Design review of the part built by this model. Coordinates are the model's own, in mm. A direction names the side the tool comes from. Give positions to 0.01 mm unless a question says otherwise; leave off trailing zeros. Write each loop counter-clockwise with the first axis right and the second up, starting at its lowest first coordinate (ties: lowest second). Pieces come first, ordered by that corner, then holes. Notation, with made-up numbers: (82.25, 76) -> (100.25, 76) arc R19 cw to (100.25, 102) -> close; hole circle Ø4 at (60, 42). An arc over 180 degrees is marked (long way). Answer as a JSON object with one key per item and string values.
```python
from build123d import *

# Parameters (mm, degrees)
SKETCH_1_R          = 2
SKETCH_1_W          = 20
SKETCH_1_H          = 50
EXTRUDE_1_DEPTH     = 3
FILLET_1_R          = 40
SKETCH_2_R          = 2
CUT_EXTRUDE_1_DEPTH = 10


with BuildPart() as part:
    # 草图1 → 凸台-拉伸1 (new body)
    # profile 1 of 3: a face of its own
    with BuildSketch(Plane.XY):
        Polygon((10, 36.547005384), (-10, 25), (10, 25), align=None)
    # profile 2 of 3: a face of its own
    with BuildSketch(Plane.XY):
        Polygon((20.980762114, 65.980762114), (30.980762114, 48.660254038), (-20.980762114, 18.660254038), (-30.980762114, 35.980762114), align=None)
        with Locations((0, 42.320508076)):
            Circle(SKETCH_1_R, mode=Mode.SUBTRACT)
        with Locations((17.320508076, 52.320508076)):
            Circle(SKETCH_1_R, mode=Mode.SUBTRACT)
        with Locations((-17.320508076, 32.320508076)):
            Circle(SKETCH_1_R, mode=Mode.SUBTRACT)
    # profile 3 of 3: a face of its own
    with BuildSketch(Plane.XY):
        Rectangle(SKETCH_1_W, SKETCH_1_H)
    extrude(amount=EXTRUDE_1_DEPTH)

    # 圆角1
    # the kernel refuses this fillet: 40 mm, written as the material it adds along each edge
    with BuildSketch(Plane(origin=(10, 36.547005384, 0), x_dir=(0, -1, 0), z_dir=(0, 0, 1))) as fillet_1_piece_1:
        with BuildLine():
            CenterArc((FILLET_1_R * 0.57735026919, FILLET_1_R), FILLET_1_R, 210, 60)
            Line((-FILLET_1_R * 0.288675134595, FILLET_1_R * 0.5), (-FILLET_1_R * 0.305995642671, FILLET_1_R * 0.49))
            Line((-FILLET_1_R * 0.305995642671, FILLET_1_R * 0.49), (-FILLET_1_R * 0.0115470053838, -FILLET_1_R * 0.02))
            Line((-FILLET_1_R * 0.0115470053838, -FILLET_1_R * 0.02), (FILLET_1_R * 0.57735026919, -FILLET_1_R * 0.02))
            Line((FILLET_1_R * 0.57735026919, -FILLET_1_R * 0.02), (FILLET_1_R * 0.57735026919, 0))
        make_face()
    extrude(amount=3)
    with BuildSketch(Plane(origin=(-10, 25, 0), x_dir=(-0.8660254037844363, -0.5000000000000041, 0), z_dir=(0, 0, 1))) as fillet_1_piece_2:
        with BuildLine():
            CenterArc((51.575734141, 9.331791971), FILLET_1_R, 150, 43.49112832)
            Line((16.93471799, 29.331791971), (16.241897667, 29.731791971))
            Line((16.241897667, 29.731791971), (-0.692820323, 0.4))
            Line((-0.692820323, 0.4), (0, -0.8))
            ThreePointArc((0, -0.8), (6.339745962, -0.8), (11.90156708, -0.186635839))
            Line((11.90156708, -0.186635839), (12.679491924, 0))
        make_face()
    extrude(amount=3)

    # 草图2 → 切除-拉伸1 (cut)
    with BuildSketch(Plane(origin=(0, 0, 0), x_dir=(-1, 0, 0), z_dir=(0, 0, -1))):
        with Locations((0, 9.601800669)):
            Circle(SKETCH_2_R)
        with Locations((0, -10.398199331)):
            Circle(SKETCH_2_R)
    extrude(amount=-CUT_EXTRUDE_1_DEPTH, mode=Mode.SUBTRACT)


solid = part.part
```
(1) Clearance check with flat-ended pins moving along their axes: pin 1 (0.9 mm diameter, centred on y = -7, z = 2, fed in from +X); pin 2 (2 mm diameter, centred on x = -11, y = -6, fed in from -Z); pin 3 (1.5 mm diameter, centred on y = -13, z = 1, fed in from -X); pin 4 (1 mm diameter, centred on y = 17, z = 1.5, fed in from +X). State where each tip first meets the part, or that it passes through.
Here are the results:
{"pin 1": "stops at x = 10", "pin 2": "stops at z = 0", "pin 3": "stops at x = -10", "pin 4": "stops at x = 10.21"}
(2) The part is to be moulded in two halves that separate along X. For faces 1 (the cylindrical face through (-16.25, 34.01, 1.48)), 2 (the flat face through (25.91, 57.44, 1.48)), 3 (the flat face through (4, 23, 0)), say which applies: +X half, -X half, draft (parallel to the pull), parting line (faces both ways), or undercut.
Here are the results:
{"face 1": "undercut", "face 2": "+X half", "face 3": "draft"}
(3) We need section C-C, the plane y = -6.5. State the section outline as (x, z) points.
Here are the results:
{"outline": "(-10.07, 0) -> (10, 0) -> (10, 3) -> (-10.07, 3) -> close"}
(4) We need section A-A, the plane x = 0. State the section outline as (y, z) points, then the cut area to 3 significant figures.
Here are the results:
{"outline": "(-25, 0) -> (-12.4, 0) -> (-12.4, 3) -> (-25, 3) -> close; (-8.4, 0) -> (7.6, 0) -> (7.6, 3) -> (-8.4, 3) -> close; (11.6, 0) -> (40.32, 0) -> (40.32, 3) -> (11.6, 3) -> close; (44.32, 0) -> (53.87, 0) -> (53.87, 3) -> (44.32, 3) -> close", "area": "201 mm²"}
(5) For line 1 along Y through (x, z) = (0, 0.7); line 2 along X through (y, z) = (-14, 0.7); line 3 along X through (y, z) = (43.5, 0.7), list the stretches that pass through material, from the lowest coordinate up.
Here are the results:
{"line 1": "y = -25 to -12.4, -8.4 to 7.6, 11.6 to 40.32, 44.32 to 53.87", "line 2": "x = -10 to 10", "line 3": "x = -17.96 to -1.62, 1.62 to 23.6"}
(6) We need section D-D, the plane y = 6. State the section outline as (x, z) points, then the cut area to 3 significant figures.
Here are the results:
{"outline": "(-12.87, 0) -> (10, 0) -> (10, 3) -> (-12.87, 3) -> close", "area": "68.6 mm²"}
(7) We need section B-B, the plane z = 1. State the section outline as (x, y) points, then the cut area to 3 significant figures.
Here are the results:
{"outline": "(-30.98, 35.98) -> (-20.98, 18.66) arc R40 cw to (-10, -8.87) -> (-10, -25) -> (10, -25) -> (10, 13.45) arc R40 cw to (30, 48.09) -> (30.98, 48.66) -> (20.98, 65.98) -> close; hole circle Ø4 at (-17.32, 32.32); hole circle Ø4 at (0, -10.4); hole circle Ø4 at (0, 9.6); hole circle Ø4 at (0, 42.32); hole circle Ø4 at (17.32, 52.32)", "area": "2,470 mm²"}
(8) For faces 4 (the flat face through (10, -6, 1)), 5 (the cylindrical face through (-0.26, 44.303, 1.479)), 6 (the flat face through (-10, -17, 1)), list the 3-axis set-ups (+Z, -Z, +X, -X, +Y, -Y) from which the entire face can be reached by the end or side of a thin tool; tool diameter is ignored.
Here are the results:
{"face 4": "+Z, -Z, +X, -Y", "face 5": "+Z, -Z", "face 6": "+Z, -Z, -X, -Y"}
